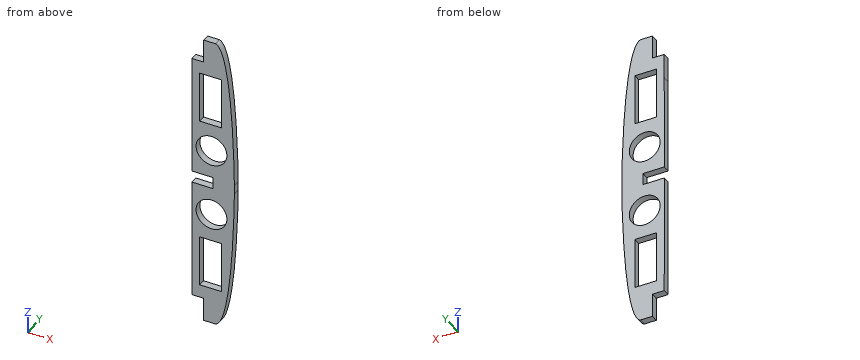
```python
from build123d import *

# Parameters (mm, degrees)
F0_R     = 13.033720186
F0_W     = 18.248938024
F0_H     = 43.4933193028
F1_DEPTH = 6


# Not quite as in the source:
# - a feature names something its author has since deleted; it is built from what else it names


with BuildPart() as f1:
    # F0 (on Front) → F1 (new body)
    with BuildSketch(Plane.XZ):
        with BuildLine():
            add(Edge.make_bspline(
                [(105.1375677345, 103.5958733921), (118.915635106, 100.3235823913), (120.9318600426, 1.7429371205), (121.1375677345, -19.7457277863)],
                knots=[0, 0, 0, 0, 110.2279027072, 110.2279027072, 110.2279027072, 110.2279027072], degree=3))
            Line((105.1375677345, 103.5958733921), (95.2585982296, 103.5958733921))
            Line((95.2585982296, 103.5958733921), (95.2585982296, 83.5958733921))
            Line((95.2585982296, 83.5958733921), (85.2585982296, 83.5958733921))
            Line((85.2585982296, 83.5958733921), (85.2585982296, 62.4470586631))
            Line((85.2585982296, 62.4470586631), (85.1375677345, -18.4041266079))
            Line((85.1375677345, -18.4041266079), (103.1375677345, -18.4041266079))
            Line((103.1375677345, -18.4041266079), (103.1375677345, -23.4041266079))
            Line((103.1375677345, -23.4041266079), (121.1375677345, -23.4041266079))
            Line((121.1375677345, -23.4041266079), (121.1375677345, -19.7457277863))
        make_face()
        with Locations((101.7788599941, 5.3969110339)):
            Circle(F0_R, mode=Mode.SUBTRACT)
        with Locations((100.9382642806, 50.7787894458)):
            Rectangle(F0_W, F0_H, mode=Mode.SUBTRACT)
        with BuildLine():
            Line((121.1375677345, -27.0625254295), (121.1375677345, -23.4041266079))
            Line((121.1375677345, -23.4041266079), (103.1375677345, -23.4041266079))
            Line((103.1375677345, -23.4041266079), (103.1375677345, -28.4041266079))
            Line((103.1375677345, -28.4041266079), (85.1375677345, -28.4041266079))
            Line((85.1375677345, -28.4041266079), (85.2585982296, -130.4041266079))
            Line((85.2585982296, -130.4041266079), (95.2585982296, -130.4041266079))
            Line((95.2585982296, -130.4041266079), (95.2585982296, -150.4041266079))
            Line((95.2585982296, -150.4041266079), (105.1375677345, -150.4041266079))
            add(Edge.make_bspline(
                [(105.1375677345, -150.4041266079), (118.915635106, -147.1318356072), (120.9318600426, -48.5511903363), (121.1375677345, -27.0625254295)],
                knots=[0, 0, 0, 0, 110.2279027072, 110.2279027072, 110.2279027072, 110.2279027072], degree=3))
        make_face()
        with Locations((100.9382642806, -97.5870426616)):
            Rectangle(F0_W, F0_H, mode=Mode.SUBTRACT)
        with Locations((101.7788599941, -52.2051642497)):
            Circle(F0_R, mode=Mode.SUBTRACT)
    extrude(amount=F1_DEPTH)


solid = f1.part
```
Can you work these out from the model? Positions are in its coordinate system, mm. Give positions to 0.01 mm unless a question says otherwise; leave off trailing zeros. Loops run counter-clockwise (first coordinate to the right, second up) from the corner with the lowest first, then second, coordinate; pieces in that order, holes last. Notation, with made-up numbers: M 38,67.5 L 71,67.5 A16 cw 71,89.5 Z; hole C 15,19 d11. An arc over 180 degrees is marked long. Use one line per item in the form item = value. Start each with the question number.
(1) Please list where these lines run through material, in increasing order: line 1 (Z direction, x = 101, y = -4); line 2 (Z direction, x = 94, y = -0.75); line 3 (Z direction, x = 91, y = -5.5).
(2) I want a section at B-B, the plane y = -4.5. State how many separate pieces and enclosed holes the cut face has, and give its area (3 significant figures).
(3) I'm going to push flat-ended pins straight in: P1, Ø3, axis at y = -3, z = -107, coming from the +X side; P2, Ø6, axis at x = 106, z = -122, coming from the +Y side; P3, Ø21, axis at x = 101.78, z = -52.21, coming from the -Y side; P4, Ø1.8, axis at x = 89, y = -2.5, coming from the +Z side. Where does each tip first touch, or does it pass through?
(4) I want a section at A-A, the plane x = 98. Write out the boundary of the cut face in (y, z).
Worked out:
q1.line_1 = -150.4 to -119.33, -75.84 to -65.22, -39.19 to -28.4, -18.4 to -7.61, 18.41 to 29.03, 72.53 to 103.6
q1.line_2 = -130.4 to -119.33, -75.84 to -62.66, -41.75 to -28.4, -18.4 to -5.06, 15.85 to 29.03, 72.53 to 83.6
q1.line_3 = -130.4 to -59.53, -44.88 to -28.4, -18.4 to -1.93, 12.72 to 83.6
q2.separate_pieces = 1
q2.enclosed_holes = 4
q2.area = 5,010 mm²
q3.P1 = 117.33
q3.P2 = 0
q3.P3 = through
q3.P4 = 83.6
q4.outline = M -6,-150.4 L 0,-150.4 L 0,-119.33 L -6,-119.33 Z; M -6,-75.84 L 0,-75.84 L 0,-64.68 L -6,-64.68 Z; M -6,-39.73 L 0,-39.73 L 0,-28.4 L -6,-28.4 Z; M -6,-18.4 L 0,-18.4 L 0,-7.08 L -6,-7.08 Z; M -6,17.87 L 0,17.87 L 0,29.03 L -6,29.03 Z; M -6,72.53 L 0,72.53 L 0,103.6 L -6,103.6 Z
